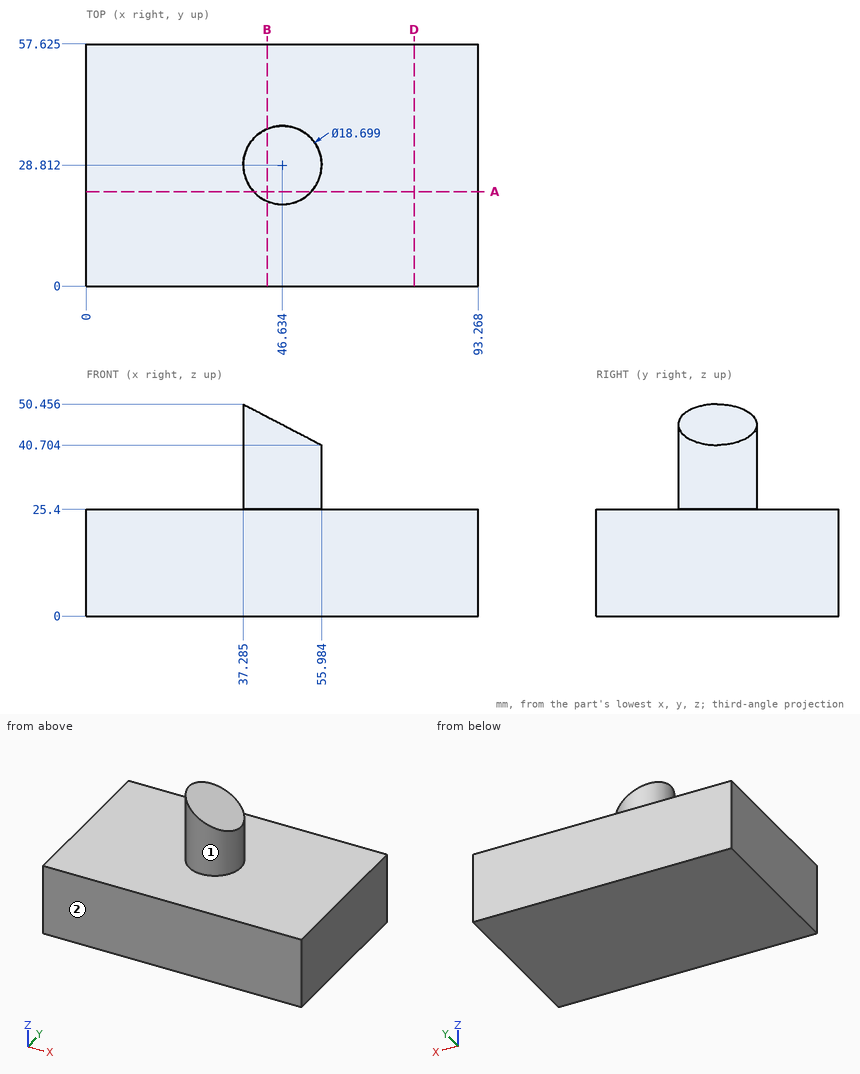
Geometry check sheet. Reference: drawing and pictorial views, mm from the part's lowest x, y, z. A direction names the side the tool comes from. Coordinates: 2 decimals unless noted, no trailing zeros. Write each loop counter-clockwise with the first axis right and the second up, starting at its lowest first coordinate (ties: lowest second). Pieces come first, ordered by that corner, then holes. Notation, with made-up numbers: (-6, 40.25) -> (30, 40.25) arc R14 ccw to (30, 44.25) -> close; hole circle Ø6 at (-7, 86). An arc over 180 degrees is marked (long way). Use a Markdown table: item, result.
1. Sectioned sample at D-D (x = 78). Enter the section's corners in (y, z) (1 decimal).
Reported:
| item | result |
|---|---|
| outline | (0, 0) -> (57.6, 0) -> (57.6, 25.4) -> (0, 25.4) -> close |
2. Go/stop test with flat-tipped pins: pin 1 Ø1.5 at (x, y) = (64, 27.5) entering from -Z; pin 2 Ø6 at (x, y) = (31, 25) entering from +Z. Record where each tip stops, or that it passes through.
Reported:
| item | result |
|---|---|
| pin 1 | stops at z = 0 |
| pin 2 | stops at z = 25.4 |
3. Sectioned sample at B-B (x = 43). Enter the section's corners in (y, z) (1 decimal), plus the area to 3 significant figures.
Reported:
| item | result |
|---|---|
| outline | (0, 0) -> (57.6, 0) -> (57.6, 25.4) -> (37.4, 25.4) -> (37.4, 47.5) -> (20.2, 47.5) -> (20.2, 25.4) -> (0, 25.4) -> close |
| area | 1,840 mm2 |
4. Sectioned sample at A-A (y = 22.5). Enter the section's corners in (x, z).
Reported:
| item | result |
|---|---|
| outline | (0, 0) -> (93.27, 0) -> (93.27, 25.4) -> (53.53, 25.4) -> (53.53, 41.98) -> (39.74, 49.18) -> (39.74, 25.4) -> (0, 25.4) -> close |
5. Scan lines: line 1 along Z through (x, y) = (84, 23.5); line 2 along X through (y, z) = (31, 38.5) (1 decimal); line 3 along X through (y, z) = (21.5, 48) (1 decimal). Record each from-to range of solid material in increasing order.
Reported:
| item | result |
|---|---|
| line 1 | z = 0 to 25.4 |
| line 2 | x = 37.5 to 55.7 |
| line 3 | x = 40.8 to 42 |
6. Tool access check on the marked faces 1 and 2. Record the directions out of +Z, -Z, +X, -X, +Y, -Y that give a thin tool (end or side, any length) a straight path to the whole face; none if there is none.
Reported:
| item | result |
|---|---|
| face 1 | +Z |
| face 2 | +Z, -Z, +X, -X, -Y |
